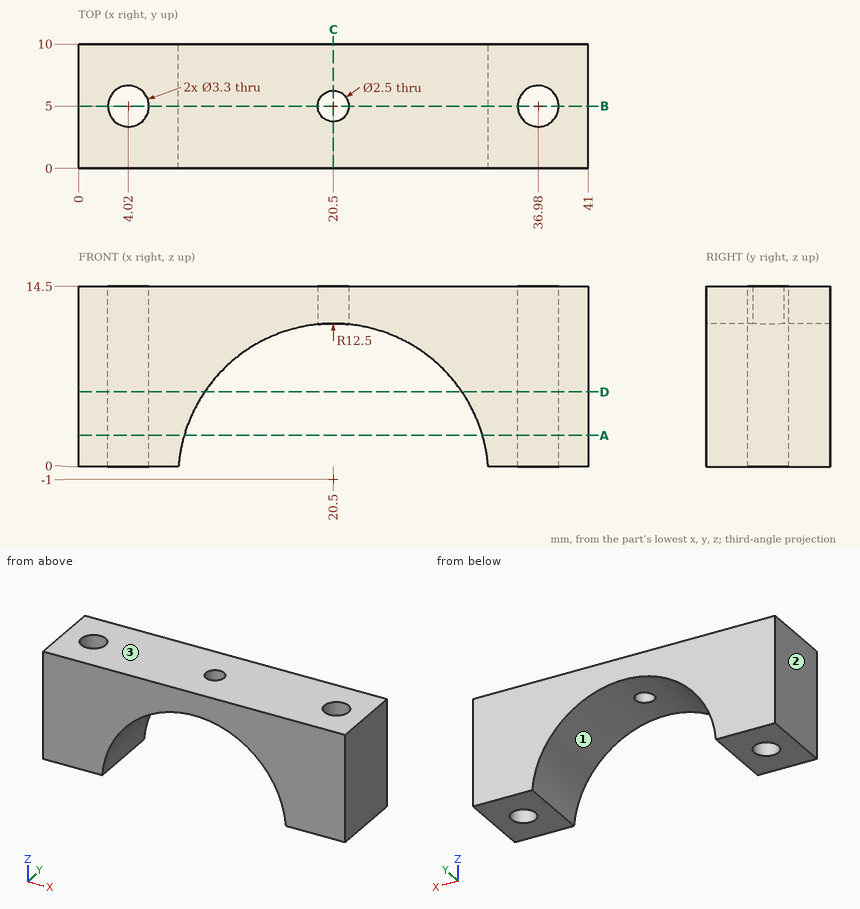
Could you check a few things on this drawing? It's one solid part, dimensions in mm from its lowest x, y, z. Coordinates: 2 decimals unless noted, no trailing zeros. Write each loop counter-clockwise with the first axis right and the second up, starting at its lowest first coordinate (ties: lowest second). Pieces come first, ordered by that corner, then holes. Notation, with made-up numbers: M 36,68.25 L 64,68.25 A21 ccw 64,103.25 Z; hole C 40,-12 d11. An arc over 180 degrees is marked long. One line per question, with ' | ' between items.
1) Imagine slicing it at C-C, the plane x = 20.5. Write out the boundary of the cut face in (y, z).
Checks:
outline: M 0,11.5 L 3.75,11.5 L 3.75,14.5 L 0,14.5 Z; M 6.25,11.5 L 10,11.5 L 10,14.5 L 6.25,14.5 Z
2) Imagine slicing it at A-A, the plane z = 2.5. Write out the boundary of the cut face in (x, y).
Checks:
outline: M 0,0 L 8.5,0 L 8.5,10 L 0,10 Z; M 32.5,0 L 41,0 L 41,10 L 32.5,10 Z; hole C 4.02,5 d3.3; hole C 36.98,5 d3.3
3) Imagine slicing it at D-D, the plane z = 6. Write out the boundary of the cut face in (x, y).
Checks:
outline: M 0,0 L 10.14,0 L 10.14,10 L 0,10 Z; M 30.86,0 L 41,0 L 41,10 L 30.86,10 Z; hole C 4.02,5 d3.3; hole C 36.98,5 d3.3
4) For pin 1 Ø2 at (x, y) = (20.5, 5) entering from +Z; pin 2 Ø1.5 at (x, y) = (25, 7.5) entering from -Z, each with a flat end and sliding along its axis, tell me the tip position at first contact or that it passes through.
Checks:
pin 1: through | pin 2: z = 10.34
5) If we mould it in two halves opening along X, with no side actions, what happens to the marked faces 1, 2 and 3? For each: released by +X, released by -X, zero draft, split by the parting line, or undercut.
Checks:
face 1: undercut | face 2: released by -X | face 3: zero draft
6) I need wall thicknesses on probe 1 along Y at (x, z) = (20.5, 13.4); probe 2 along X at (y, z) = (5.5, 0.75); probe 3 along X at (y, z) = (5.75, 7.5) (1 decimal). Which ranges of each line are inside material? Lowest first, please. Write a range as [from, to].
Checks:
probe 1: [0, 3.75], [6.25, 10] | probe 2: [0, 2.45], [5.59, 8.12], [32.88, 35.41], [38.55, 41] | probe 3: [0, 2.6], [5.5, 11.3], [29.7, 35.5], [38.4, 41]
7) Imagine slicing it at B-B, the plane y = 5. Write out the boundary of the cut face in (x, z).
Checks:
outline: M 0,0 L 2.37,0 L 2.37,14.5 L 0,14.5 Z; M 5.67,0 L 8.04,0 A12.5 cw 19.25,11.44 L 19.25,14.5 L 5.67,14.5 Z; M 21.75,11.44 A12.5 cw 32.96,0 L 35.33,0 L 35.33,14.5 L 21.75,14.5 Z; M 38.63,0 L 41,0 L 41,14.5 L 38.63,14.5 Z
